Model file for the job. Use its own axes, mm. Round coordinates to 2 decimals unless told otherwise and drop trailing zeros. Loops run counter-clockwise (first coordinate to the right, second up) from the corner with the lowest first, then second, coordinate; pieces in that order, holes last. Notation, with made-up numbers: M 79,-5.75 L 99,-5.75 A24 ccw 99,20.25 Z; hole C 29,-2 d10. An arc over 180 degrees is marked long. Answer in a Markdown table with one row per item.
from build123d import *

# Parameters (mm, degrees)
ESQUISSE1_W                  = 80
ESQUISSE1_H                  = 125
BOSS_EXTRU_1_DEPTH           = 9
ESQUISSE2_W                  = 20
ESQUISSE2_H                  = 9
ENL_V_MAT_EXTRU_1_DEPTH      = 9
ENL_V_MAT_EXTRU_2_DEPTH      = 149.680866287
ENL_V_MAT_EXTRU_2_DEPTH_BACK = 149.680866287
ESQUISSE3_R                  = 1.65
ESQUISSE4_R                  = 1.65
ENL_V_MAT_EXTRU_3_DEPTH      = 9


with BuildPart() as part:
    # Esquisse1 → Boss.-Extru.1 (new body)
    with BuildSketch(Plane.XY):
        with Locations((40, 62.5)):
            Rectangle(ESQUISSE1_W, ESQUISSE1_H)
    extrude(amount=BOSS_EXTRU_1_DEPTH)

    # Esquisse2 → Enlèv. mat.-Extru.1 (cut)
    with BuildSketch(Plane.XY.offset(9)):
        with Locations((17, 7)):
            Rectangle(ESQUISSE2_W, ESQUISSE2_H)
        with Locations((63, 118)):
            Rectangle(ESQUISSE2_W, ESQUISSE2_H)
    extrude(amount=-ENL_V_MAT_EXTRU_1_DEPTH, mode=Mode.SUBTRACT)

    # Esquisse3 → Enlèv. mat.-Extru.2 (cut, two sides: drawn at the far end of the back side and taken through both)
    with BuildSketch(Plane.XY.offset(9).offset(-ENL_V_MAT_EXTRU_2_DEPTH_BACK)):
        with Locations((3.5, 7)):
            Circle(ESQUISSE3_R)
        with Locations(Location((30.5, 7, 0), (0, 0, 180))):
            Circle(ESQUISSE3_R)
        with Locations(Location((49.5, 118, 0), (0, 0, 180))):
            Circle(ESQUISSE3_R)
        with Locations((76.5, 118)):
            Circle(ESQUISSE3_R)
        with BuildLine():
            Line((7, 9.025126266), (9.474873734, 11.5))
            ThreePointArc((9.474873734, 11.5), (6.929289322, 11.570710678), (7, 9.025126266))
        make_face()
        with BuildLine():
            Line((27, 9.025126266), (24.525126266, 11.5))
            ThreePointArc((24.525126266, 11.5), (27.070710678, 11.570710678), (27, 9.025126266))
        make_face()
        with BuildLine():
            Line((27, 4.974873734), (24.525126266, 2.5))
            ThreePointArc((24.525126266, 2.5), (27.070710678, 2.429289322), (27, 4.974873734))
        make_face()
        with BuildLine():
            Line((7, 4.974873734), (9.474873734, 2.5))
            ThreePointArc((9.474873734, 2.5), (6.929289322, 2.429289322), (7, 4.974873734))
        make_face()
        with BuildLine():
            Line((73, 115.974873734), (70.525126266, 113.5))
            ThreePointArc((70.525126266, 113.5), (73.070710678, 113.429289322), (73, 115.974873734))
        make_face()
        with BuildLine():
            Line((53, 115.974873734), (55.474873734, 113.5))
            ThreePointArc((55.474873734, 113.5), (52.929289322, 113.429289322), (53, 115.974873734))
        make_face()
        with BuildLine():
            Line((53, 120.025126266), (55.474873734, 122.5))
            ThreePointArc((55.474873734, 122.5), (52.929289322, 122.570710678), (53, 120.025126266))
        make_face()
        with BuildLine():
            Line((73, 120.025126266), (70.525126266, 122.5))
            ThreePointArc((70.525126266, 122.5), (73.070710678, 122.570710678), (73, 120.025126266))
        make_face()
    extrude(amount=ENL_V_MAT_EXTRU_2_DEPTH + ENL_V_MAT_EXTRU_2_DEPTH_BACK, mode=Mode.SUBTRACT)

    # Esquisse4 → Enlèv. mat.-Extru.3 (cut)
    with BuildSketch(Plane.XY.offset(9)):
        with Locations((7, 95)):
            Circle(ESQUISSE4_R)
        with Locations(Location((27, 95, 0), (0, 0, 180))):
            Circle(ESQUISSE4_R)
        with Locations((27, 75)):
            Circle(ESQUISSE4_R)
        with Locations(Location((7, 75, 0), (0, 0, 180))):
            Circle(ESQUISSE4_R)
        with Locations((73, 30)):
            Circle(ESQUISSE4_R)
        with Locations(Location((53, 30, 0), (0, 0, 180))):
            Circle(ESQUISSE4_R)
        with Locations((53, 50)):
            Circle(ESQUISSE4_R)
        with Locations(Location((73, 50, 0), (0, 0, 180))):
            Circle(ESQUISSE4_R)
    extrude(amount=-ENL_V_MAT_EXTRU_3_DEPTH, mode=Mode.SUBTRACT)


solid = part.part
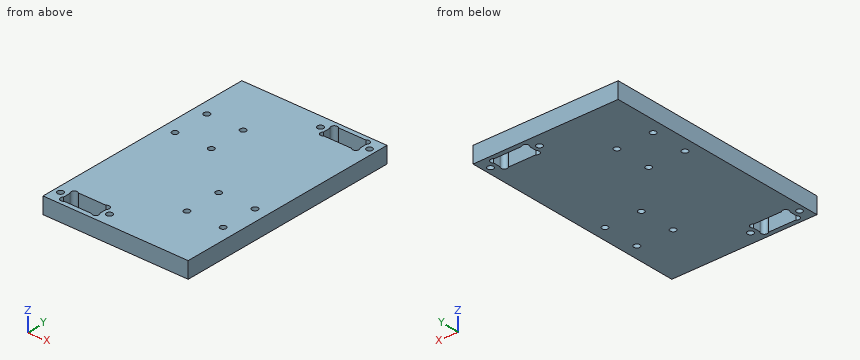
1. Wall check: probe 1 along X at (y, z) = (75, 3); probe 2 along Y at (x, z) = (5.5, 2.25); probe 3 along Y at (x, z) = (8, 8.75). Give the ranges that are in metal, low to high.
Verdict:
| item | result |
|---|---|
| probe 1 | x = 0 to 5.35, 8.65 to 25.35, 28.65 to 80 |
| probe 2 | y = 0 to 74.31, 75.69 to 94.31, 95.69 to 125 |
| probe 3 | y = 0 to 1.92, 12.08 to 73.69, 76.31 to 93.69, 96.31 to 125 |
2. Saw through at D-D (y = 118). Write the cut outline in (x, z), and give its area (3 significant figures).
Verdict:
| item | result |
|---|---|
| outline | M 0,0 L 47.85,0 L 47.85,9 L 0,9 Z; M 51.15,0 L 53,0 L 53,9 L 51.15,9 Z; M 73,0 L 74.85,0 L 74.85,9 L 73,9 Z; M 78.15,0 L 80,0 L 80,9 L 78.15,9 Z |
| area | 481 mm² |
3. Saw through at B-B (z = 7.75). State how many separate pieces and enclosed holes the cut face has, and give its area (3 significant figures).
Verdict:
| item | result |
|---|---|
| separate pieces | 1 |
| enclosed holes | 14 |
| area | 9,520 mm² |
4. Saw through at A-A (y = 95). Write the cut outline in (x, z).
Verdict:
| item | result |
|---|---|
| outline | M 0,0 L 5.35,0 L 5.35,9 L 0,9 Z; M 8.65,0 L 25.35,0 L 25.35,9 L 8.65,9 Z; M 28.65,0 L 80,0 L 80,9 L 28.65,9 Z |
5. Pin check, flat tips, straight feed: pin 1 (2 mm diameter, centred on x = 68.5, z = 4.5, fed in from -Y); pin 2 (2.5 mm diameter, centred on x = 49.5, y = 118, fed in from +Z). Stop position of each tip, or through.
Verdict:
| item | result |
|---|---|
| pin 1 | stops at y = 0 |
| pin 2 | passes through |
6. Saw through at C-C (x = 76.5). Write the cut outline in (y, z).
Verdict:
| item | result |
|---|---|
| outline | M 0,0 L 116.35,0 L 116.35,9 L 0,9 Z; M 119.65,0 L 125,0 L 125,9 L 119.65,9 Z |
